Geometry check sheet. Reference: drawing and pictorial views, mm from the part's lowest x, y, z. A direction names the side the tool comes from. Round coordinates to 2 decimals unless told otherwise and drop trailing zeros. Order: outer loops, then holes, each group sorted by start corner. A loop starts at its lowest first (then second) coordinate and runs counter-clockwise, first axis right, second up. Notation, with made-up numbers: M -28.75,34.5 L -5.75,34.5 A23 ccw -5.75,72.5 Z; hole C 22.5,75 d5. An arc over 180 degrees is marked long. Answer as a JSON object with one key per item and string values. Group by question number.
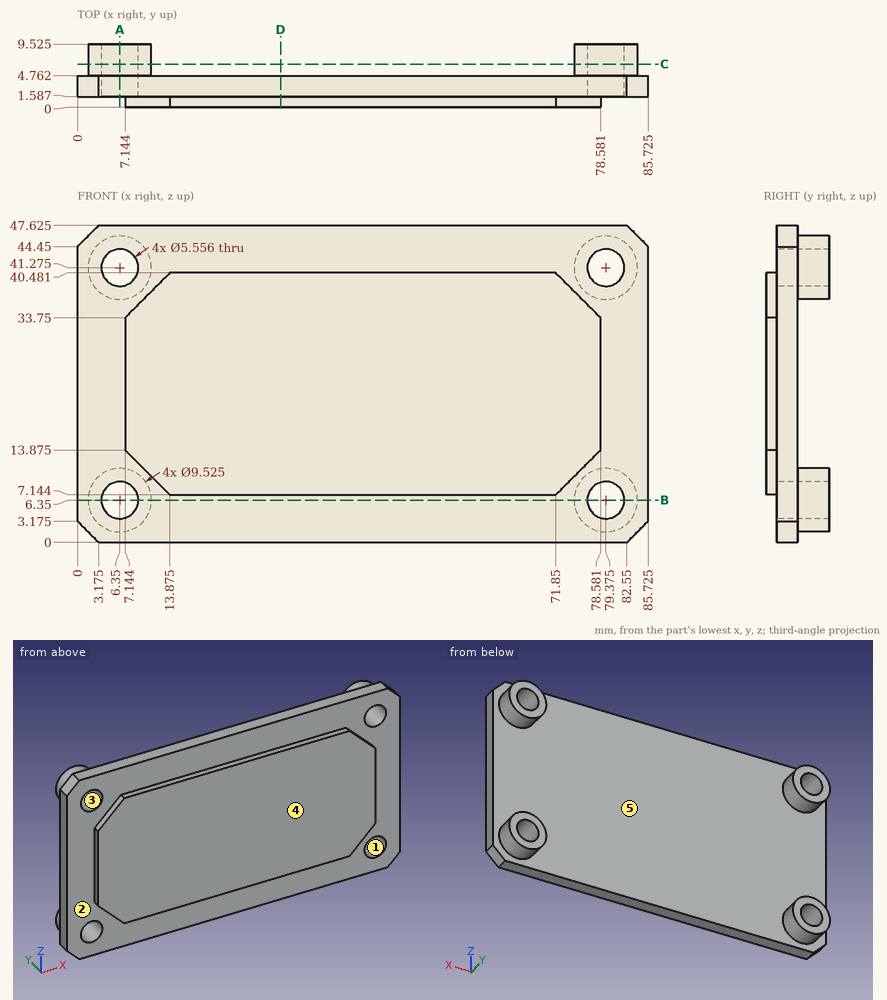
Q1. Cross-section at B-B, the plane z = 6.35. Record the cut outline in (x, y) (1 decimal).
Q2. Cross-section at C-C, the plane y = 6.5. Give the number of separate pieces and of enclosed holes in the cut face, then the cut area to 3 significant figures.
Q3. Thickness scan on line 1 (Z direction, x = 6.35, y = 7.5); line 2 (Z direction, x = 6.35, y = 3.75) (1 decimal); line 3 (X direction, y = 9, z = 39.5) (1 decimal). Record the ranges inside material, lowest first. Write a range as from..to.
Q4. Cross-section at A-A, the plane x = 6.35. Record the cut outline in (y, z) (1 decimal), then the cut area to 3 significant figures.
Q5. Gauge pin test, flat ends, axial feed: pin 1 Ø1.5 at (x, y) = (10.5, 7) entering from -Z (1 decimal); pin 2 Ø1.3 at (y, z) = (0.5, 25) entering from +X; pin 3 Ø1.5 at (x, z) = (18, 30) entering from +Y. Record the tip position at first contact, or that the pin passes through.
Q6. Tool access check on the marked faces 4 and 5. Record the directions out of +Z, -Z, +X, -X, +Y, -Y that give a thin tool (end or side, any length) a straight path to the whole face; none if there is none.
Q7. Release check for a two-part mould opening along X. For the marked faces 1, 2 and 3 record: released by +X, released by -X, zero draft, split by the parting line, or undercut.
Q8. Cross-section at D-D, the plane x = 30.5. Record the cut outline in (y, z) (1 decimal).
Conclusion:
{
 "1": {"outline": "M 0,1.6 L 3.6,1.6 L 3.6,9.5 L 1.6,9.5 L 1.6,4.8 L 0,4.8 Z; M 9.1,1.6 L 76.6,1.6 L 76.6,9.5 L 74.6,9.5 L 74.6,4.8 L 11.1,4.8 L 11.1,9.5 L 9.1,9.5 Z; M 82.2,1.6 L 85.7,1.6 L 85.7,4.8 L 84.1,4.8 L 84.1,9.5 L 82.2,9.5 Z"},
 "2": {"separate pieces": "4", "enclosed holes": "4", "area": "188 mm2"},
 "3": {"line 1": "1.59..3.57, 9.13..11.11, 36.51..38.5, 44.05..46.04", "line 2": "0..3.6, 9.1..38.5, 44.1..47.6", "line 3": "1.9..4.2, 8.5..10.8, 75..77.2, 81.5..83.8"},
 "4": {"outline": "M 1.6,0 L 4.8,0 L 4.8,1.6 L 9.5,1.6 L 9.5,3.6 L 1.6,3.6 Z; M 1.6,9.1 L 9.5,9.1 L 9.5,11.1 L 4.8,11.1 L 4.8,36.5 L 9.5,36.5 L 9.5,38.5 L 1.6,38.5 Z; M 1.6,44.1 L 9.5,44.1 L 9.5,46 L 4.8,46 L 4.8,47.6 L 1.6,47.6 Z", "area": "154 mm2"},
 "5": {"pin 1": "z = 3", "pin 2": "x = 78.58", "pin 3": "y = 4.76"},
 "6": {"face 4": "+Z, -Z, +X, -X, -Y", "face 5": "+Y"},
 "7": {"face 1": "undercut", "face 2": "zero draft", "face 3": "undercut"},
 "8": {"outline": "M 0,7.1 L 1.6,7.1 L 1.6,0 L 4.8,0 L 4.8,47.6 L 1.6,47.6 L 1.6,40.5 L 0,40.5 Z"}
}
